```python
from build123d import *

# Parameters (mm, degrees)
F4_R = 5.99999


# Not quite as in the source:
# - a fillet or chamfer is up to 0.001 mm smaller than in the source, because OpenCascade refuses the exact size


with BuildPart() as f1:
    # F0 (on Front) → F1 (revolve)
    with BuildSketch(Plane.XZ):
        with BuildLine():
            Line((0, 31), (0, 0))
            Line((0, 0), (88, 0))
            Line((88, 0), (88, 16))
            Line((88, 16), (85, 16))
            Line((85, 16), (85, 20))
            Line((85, 20), (68, 20))
            Line((68, 20), (68, 31))
            Line((68, 31), (56, 31))
            ThreePointArc((56, 31), (50, 25), (44, 31))
            Line((44, 31), (0, 31))
        make_face()
    revolve(axis=Axis((-6.5542864613, 0, 0), (-1, 0, 0)))

    # F2 (on Front) → F3 (revolve, cut)
    with BuildSketch(Plane.XZ):
        Polygon((0, 25), (0, 0), (88, 0), (88, 6), (30, 6), (30, 12.5), (22, 12.5), (22, 20.5), (15, 20.5), (15, 12.5), (12, 12.5), (12, 16), (1.5, 16), (1.5, 25), align=None)
    revolve(axis=Axis((44, 0, 0), (-1, 0, 0)), mode=Mode.SUBTRACT)

    # F4 (radius 6 in the source; OpenCascade refuses exactly that, so slightly less here)
    f4_edges = [f1.edges().sort_by_distance(p)[0] for p in [
        (0, 0, -31),
    ]]
    fillet(f4_edges, radius=F4_R)


solid = f1.part
```
Work out the finished part from the listing and answer in its coordinate system (mm). A direction names the side the tool comes from. Coordinates: 2 decimals unless noted, no trailing zeros. Write each loop counter-clockwise with the first axis right and the second up, starting at its lowest first coordinate (ties: lowest second). Pieces come first, ordered by that corner, then holes.
Q1. Find the intervals of material crossed by line 1 (Y direction, x = 42, z = 0); line 2 (X direction, y = 16.5, z = -6); line 3 (Z direction, x = 66, y = 4.5), in increasing order.
Q2. Determine the mould class of faces 5 (the face through (61.916, 30.736, -4.036)), 6 (the face through (68, -20.2, 0.4)), 7 (the face through (6.68, -15.62, -3.47)) for opening direction Z: released by +Z, released by -Z, zero draft, split by the parting line, or undercut.
Q3. A cutting plane is placed at A-A, the plane x = 66.5. Give the vertices of the cut face in (y, z), then the cut area to 3 significant figures.
Q4. Each of these flat-tipped pins is pushed along its axis until it touches: pin 1 Ø1.5 at (y, z) = (-24.5, -6) entering from +X; pin 2 Ø1 at (x, y) = (73.5, -22) entering from -Z; pin 3 Ø9.5 at (y, z) = (0, 4) entering from -X; pin 4 Ø1.5 at (x, z) = (31.5, 11) entering from +Y. Where does it stop, or does it pass through?
Q5. Which of the six approach directions +Z, -Z, +X, -X, +Y, -Y give full straight-line access (tool end or side, diameter ignored) to faces 1 (the face through (12, -8, 10)), 2 (the face through (88, 0, -7)), 3 (the face through (18.451, -20.013, -4.444)), 4 (the face through (76.381, -19.524, -4.336))?
Q6. A cutting plane is placed at B-B, the plane x = 53. Give the vertices of the cut face in (y, z), then the cut area to 3 significant figures.
Findings below:
1. line 1: y = -31 to -6, 6 to 31
1. line 2: x = 1.5 to 15, 22 to 85
1. line 3: z = -30.67 to -3.97, 3.97 to 30.67
2. face 5: split by the parting line
2. face 6: zero draft
2. face 7: undercut
3. outline: circle Ø62 at (0, 0); hole circle Ø12 at (0, 0)
3. area: 2,910 mm2
4. pin 1: stops at x = 68
4. pin 2: passes through
4. pin 3: stops at x = 30
4. pin 4: stops at y = 29.26
5. face 1: -X
5. face 2: +Z, -Z, +X, +Y, -Y
5. face 3: none
5. face 4: +X
6. outline: circle Ø51.61 at (0, 0); hole circle Ø12 at (0, 0)
6. area: 1,980 mm2
